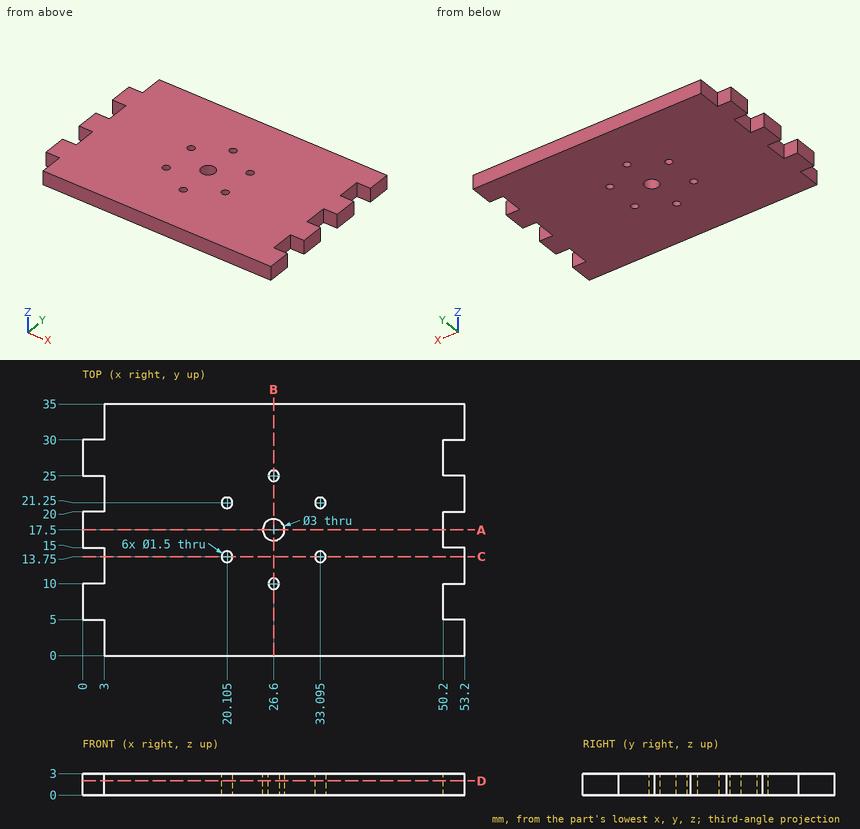
Part print with two shaded views. Sizes in mm from the minimum x, y, z corner. Round coordinates to 2 decimals unless told otherwise and drop trailing zeros. Order: outer loops, then holes, each group sorted by start corner. A loop starts at its lowest first (then second) coordinate and runs counter-clockwise, first axis right, second up. Notation, with made-up numbers: M 44.5,27.5 L 79.5,27.5 A20 cw 79.5,65.5 Z; hole C -30.75,-32 d8. An arc over 180 degrees is marked long. Put each result on its own line as item: value. Start each with the question number.
1. Drill centre lines: probe 1 along Y at (x, z) = (26.6, 1); probe 2 along X at (y, z) = (7, 0.95); probe 3 along X at (y, z) = (14, 0.15). Where is each one in solid material? Low to high. Write a range as [from, to].
2. Slice it at C-C on y = 13.75. List the corners of the cut face in (x, z) (1 decimal), then the cut area to 3 significant figures.
3. Drop flat-ended pins along their axis: pin 1 (0.9 mm diameter, centred on y = 28, z = 2, fed in from +X); pin 2 (1.5 mm diameter, centred on y = 33.5, z = 1, fed in from -X). Give the stop position or say it passes through.
4. Slice it at B-B on x = 26.6. List the corners of the cut face in (y, z).
5. Slice it at D-D on z = 2. State how many separate pieces and enclosed holes the cut face has, then the cut area to 3 significant figures.
6. Slice it at A-A on y = 17.5. List the corners of the cut face in (x, z).
Findings:
1. probe 1: [0, 9.25], [10.75, 16], [19, 24.25], [25.75, 35]
1. probe 2: [0, 50.2]
1. probe 3: [3, 19.4], [20.81, 32.39], [33.8, 53.2]
2. outline: M 3,0 L 19.4,0 L 19.4,3 L 3,3 Z; M 20.9,0 L 32.3,0 L 32.3,3 L 20.9,3 Z; M 33.8,0 L 53.2,0 L 53.2,3 L 33.8,3 Z
2. area: 142 mm2
3. pin 1: x = 50.2
3. pin 2: x = 3
4. outline: M 0,0 L 9.25,0 L 9.25,3 L 0,3 Z; M 10.75,0 L 16,0 L 16,3 L 10.75,3 Z; M 19,0 L 24.25,0 L 24.25,3 L 19,3 Z; M 25.75,0 L 35,0 L 35,3 L 25.75,3 Z
5. separate pieces: 1
5. enclosed holes: 7
5. area: 1,740 mm2
6. outline: M 0,0 L 25.1,0 L 25.1,3 L 0,3 Z; M 28.1,0 L 50.2,0 L 50.2,3 L 28.1,3 Z
